from build123d import *

# Parameters (mm, degrees)
F0_W     = 28.575
F0_H     = 25.4
F1_DEPTH = 12.7
F2_W     = 23.8125
F2_H     = 14.2875
F3_DEPTH = 12.701
F5_D     = 6.7564
F5_DEPTH = 3.96875
F5_TIP   = 2.0298273432
F7_D     = 2.794


with BuildPart() as f1:
    # F0 (on Front) → F1 (new body)
    with BuildSketch(Plane.XZ):
        Rectangle(F0_W, F0_H)
    extrude(amount=F1_DEPTH)

    # F2 (on face) → F3 (cut, through all)
    with BuildSketch(Plane.XZ.offset(12.7)):
        Rectangle(F2_W, F2_H)
    extrude(amount=-F3_DEPTH, mode=Mode.SUBTRACT)

    # F5
    with Locations(Plane.YZ.offset(14.2875)):
        with Locations((-6.35, 0)):
            Hole(F5_D / 2, depth=F5_DEPTH)
            with Locations((0, 0, -(F5_DEPTH + F5_TIP / 2))):  # 118° drill point
                Cone(0, F5_D / 2, F5_TIP, mode=Mode.SUBTRACT)

    # F7 (through all)
    with Locations(Plane.XZ.offset(12.7)):
        with Locations((-9.525, 9.525), (9.525, 9.525), (9.525, -9.525), (-9.525, -9.525)):
            Hole(F7_D / 2)


solid = f1.part
Could you check a few things on this model? Use its own coordinates, in mm. A direction names the side the tool comes from. Round coordinates to 2 decimals unless told otherwise and drop trailing zeros. Loops run counter-clockwise (first coordinate to the right, second up) from the corner with the lowest first, then second, coordinate; pieces in that order, holes last. Notation, with made-up numbers: (-31.5, -26.75) - (2.5, -26.75) arc R21 cw to (2.5, -7.75) - close; hole circle Ø1 at (-3, 12). An arc over 180 degrees is marked (long way). Write item = value, one per line.
1) On a 3-axis mill with a long thin cutter (end or side, diameter ignored), from which of +Z, -Z, +X, -X, +Y, -Y can I reach the whole of each face in a straight line? I mean faces 4 (the flat face through (0, -6, -12.7)), 5 (the cylindrical face through (13.08, -9.572, 1.015)), 6 (the flat face through (0, -6, -7.144)). Say none if no direction works.
Computed:
face_4 = -Z, +X, -X, +Y, -Y
face_5 = +X
face_6 = +Y, -Y
2) Imagine slicing it at C-C (z = -6). Please give me the cut outline in (x, y).
Computed:
outline = (-14.29, -12.7) - (-11.91, -12.7) - (-11.91, 0) - (-14.29, 0) - close; (11.91, -12.7) - (14.29, -12.7) - (14.29, 0) - (11.91, 0) - close
3) Imagine slicing it at A-A (x = -3.75). Please give me the cut outline in (y, z).
Computed:
outline = (-12.7, -12.7) - (0, -12.7) - (0, -7.14) - (-12.7, -7.14) - close; (-12.7, 7.14) - (0, 7.14) - (0, 12.7) - (-12.7, 12.7) - close
4) If we mould it in two halves opening along X, with no side actions, what happens to faces 1 (the flat face through (0, 0, 9)), 2 (the flat face through (14.288, -9, 3)), 3 (the cylindrical face through (-10.86, -6.26, 9.94))? For each: pulls with the +X half, pulls with the -X half, needs draft (parallel to the pull), parting line crosses it, or undercut.
Computed:
face_1 = needs draft
face_2 = pulls with the +X half
face_3 = undercut
5) Imagine slicing it at D-D (y = -7.75). Please give me the cut outline in (x, z) (1 decimal), and give its area (3 significant figures).
Computed:
outline = (-14.3, -12.7) - (14.3, -12.7) - (14.3, -3.1) - (11.9, -3.1) - (11.9, -7.1) - (-11.9, -7.1) - (-11.9, 7.1) - (11.9, 7.1) - (11.9, 3.1) - (14.3, 3.1) - (14.3, 12.7) - (-14.3, 12.7) - close; hole circle Ø2.8 at (-9.5, -9.5); hole circle Ø2.8 at (-9.5, 9.5); hole circle Ø2.8 at (9.5, -9.5); hole circle Ø2.8 at (9.5, 9.5)
area = 346 mm2
6) Imagine slicing it at B-B (z = 0). Please give me the cut outline in (x, y), and give its area (3 significant figures).
Computed:
outline = (-14.29, -12.7) - (-11.91, -12.7) - (-11.91, 0) - (-14.29, 0) - close; (11.91, -12.7) - (14.29, -12.7) - (14.29, -9.73) - (11.91, -9.73) - close; (11.91, -2.97) - (14.29, -2.97) - (14.29, 0) - (11.91, 0) - close
area = 44.4 mm2
7) I need wall thicknesses on line 1 along X through (y, z) = (-3, -4.5); line 2 along Z through (x, y) = (1.5, -9.75); line 3 along X through (y, z) = (-8.25, 10.25). Which ranges of each line are inside material? Lowest first, please. Write a range as from..to.
Computed:
line_1 = -14.29..-11.91, 11.91..14.29
line_2 = -12.7..-7.14, 7.14..12.7
line_3 = -14.29..-10.72, -8.33..8.33, 10.72..14.29
